Job drawing, mm, ordinate dimensions from the low corner. One solid piece. Give positions to 0.01 mm unless a question says otherwise; leave off trailing zeros. Order: outer loops, then holes, each group sorted by start corner. A loop starts at its lowest first (then second) coordinate and runs counter-clockwise, first axis right, second up.
Item 1: Wall check: L1, parallel to X at y = 118, z = 1406. Give the ranges that are in metal, low to high.
Item 2: Band-saw the part on B-B on z = 1132. Give the cut face in (x, y), plus the area to 4 significant figures.
Item 3: Band-saw the part on C-C on y = 77. Give the cut face in (x, z), plus the area to 3 significant figures.
Item 4: Flat gauge pins, fed straight in: P1, Ø15, axis at x = 1533, z = 1234.5, coming from the +Y side; P2, Ø12, axis at y = 139, z = 998, coming from the +X side. Where does each tip first touch, or does it go through?
Item 5: Band-saw the part on A-A on y = 446.5. Give the cut face in (x, z) (1 decimal), plus the area to 3 significant figures.
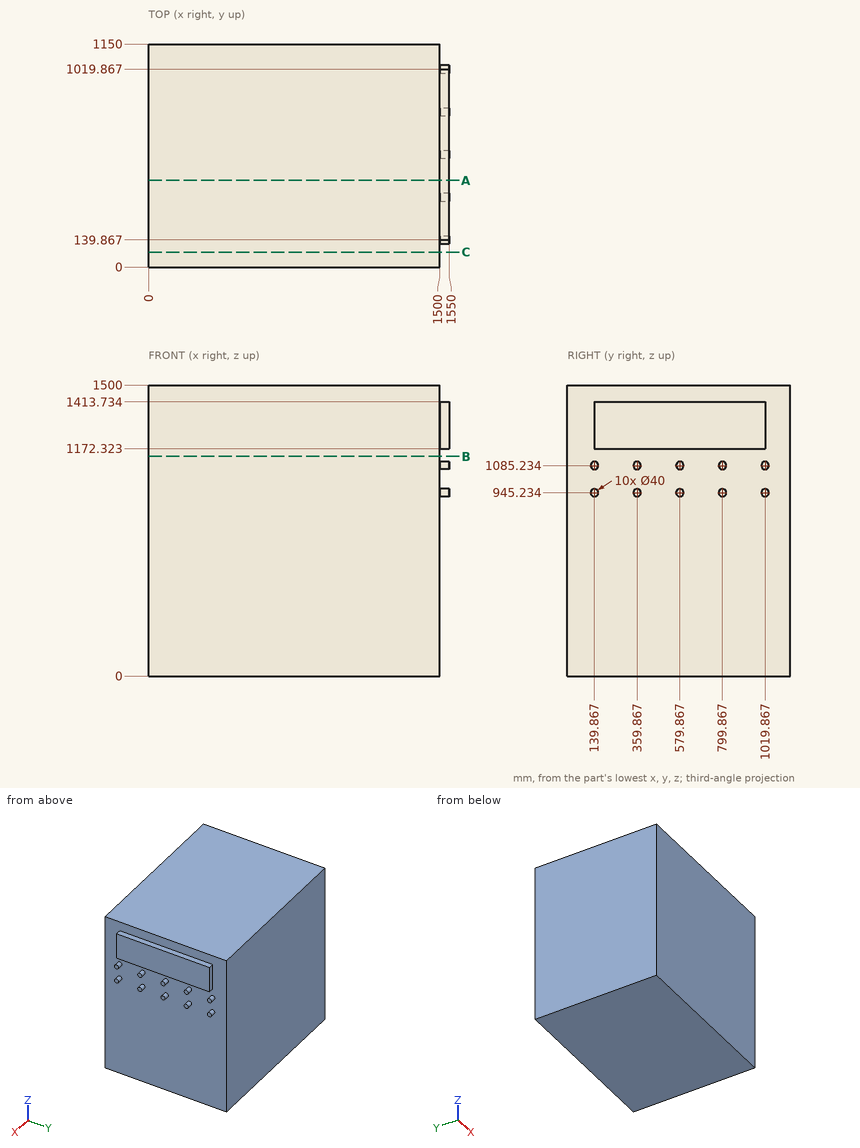
The answers:
1. L1: x = 0 to 1500
2. outline: (0, 0) - (1500, 0) - (1500, 1150) - (0, 1150) - close
2. area: 1,725,000 mm2
3. outline: (0, 0) - (1500, 0) - (1500, 1500) - (0, 1500) - close
3. area: 2,250,000 mm2
4. P1: stops at y = 1019.87
4. P2: stops at x = 1500
5. outline: (0, 0) - (1500, 0) - (1500, 1172.3) - (1550, 1172.3) - (1550, 1413.7) - (1500, 1413.7) - (1500, 1500) - (0, 1500) - close
5. area: 2,260,000 mm2
